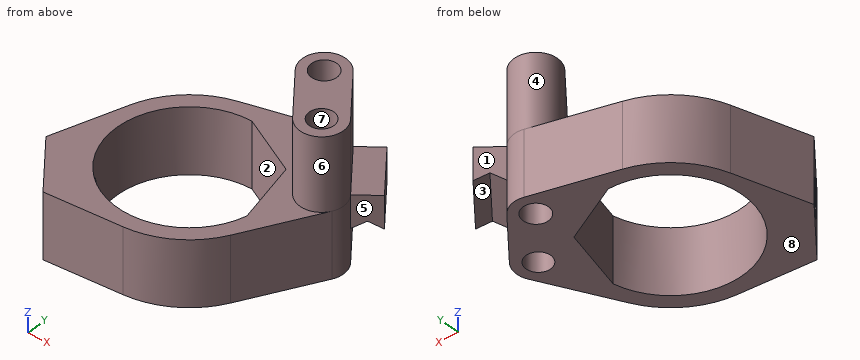
Autodesk Inventor part; units mm, degrees
ref_plane "YZ Plane" through (0, 0, 0) normal (1, 0, 0) x (0, 1, 0)
ref_plane "XZ Plane" through (0, 0, 0) normal (0, 1, 0) x (-1, 0, 0)
ref_plane "XY Plane" through (0, 0, 0) normal (0, 0, 1) x (1, 0, 0)
sketch "Sketch1" plane through (0, 0, 0) normal (0, 0, 1) x (1, 0, 0)
  circle A0 centre (83.2518, -42.1897) radius 1.5
  circle A1 centre (88.3962, -48.3162) radius 1.5
  circle A2 centre (75.2518, -54.1305) radius 10
  arc A3 (71.6612, -42.6802) -> (85.9084, -59.6473) centre (75.2518, -54.1305) ccw
  arc A4 (85.5492, -40.2605) -> (82.3541, -39.3271) centre (83.2518, -42.1897) ccw
  arc A5 (91.0604, -49.6954) -> (90.6937, -46.387) centre (88.3962, -48.3162) ccw
  line L0 (71.6612, -42.6802) -> (82.3541, -39.3271)
  line L1 (91.0604, -49.6954) -> (85.9084, -59.6473)
  line L2 (85.5492, -40.2605) -> (90.6937, -46.387)
  circle A6 centre (83.2518, -42.1897) radius 1.75
  circle A7 centre (88.3962, -48.3162) radius 1.7
  line L3 (88.1215, -43.3238) -> (66.062, -61.8472) construction
  line L4 (82.9099, -47.6999) -> (85.0453, -56.1521)
  line L5 (82.9099, -47.6999) -> (74.9544, -44.1349)
  circle A8 centre (75.2518, -54.1305) radius 9 construction
  line L6 (60.8256, -60.2763) -> (66.7035, -67.2763)
  line L7 (60.8256, -60.2763) -> (63.7758, -50.6232)
  line L8 (66.7035, -67.2763) -> (76.7214, -66.0401)
  point P0 (0, 0)
  dimension "d0" = 24
  dimension "d1" = 6
  dimension "d2" = 6
  dimension "d3" = 3.5
  dimension "d4" = 3.4
  dimension "d5" = 18
  dimension "d8" = 15
  dimension "d9" = 7
extrude "Extrusion1" add sketch "Sketch1" along normal blind 9 contours A2 L4 | L5 A2 | L0 A4 L2 A5 L1 A3 | A3 L8 L6 L7
sketch "Sketch2" plane through (66.7035, -67.2763, 0) normal (-0.7658175, -0.643058, 0) x (0, 0, 1)
  line L0 (9, 9.1406) -> (9, 0)
  line L1 (9, 4.5703) -> (0, 4.5703) construction
  line L2 (0, 9.1406) -> (0, 0)
  line L3 (0, 9.1406) -> (9, 9.1406)
  line L4 (4.5, 9.1406) -> (4.5, 0) construction
  line L5 (0, 0) -> (9, 0)
  point P0 (0, 94.4156)
  point P1 (4.5, 4.5703)
hole "Hole1" at (63.7645, -63.7763, 4.5) direction (0.7658175, 0.643058, 0) diameter 4.6 depth 8
ref_plane "Work Plane1" through (122.4886, -30.1352, -3.9205) normal (0.643058, -0.7658175, 0) x (0, 0, 1)
sketch "Sketch3" plane through (122.4886, -30.1352, -3.9205) normal (0.643058, -0.7658175, 0) x (0, 0, 1)
  line L0 (3.9205, 34.8) -> (12.9205, 34.8)
  line L1 (8.4716, 29.3) -> (8.4716, 32.8)
  line L2 (8.4716, 32.8) -> (8.4716, 33.3)
  line L3 (3.9205, 34.8) -> (12.9205, 34.8)
  line L4 (8.4716, 34.8) -> (9.4716, 33.05)
  line L5 (9.4716, 33.05) -> (8.4716, 31.3)
  line L6 (8.4716, 31.3) -> (12.9205, 31.3)
  line L7 (12.9205, 31.3) -> (12.9205, 34.8)
  line L8 (8.4716, 33.05) -> (10.4716, 33.05) construction
  point P0 (3.9205, 74.4253)
  dimension "d17" = 0.5
  dimension "d18" = 1
extrude "Extrusion2" add sketch "Sketch3" against normal blind 16
sketch "Sketch4" plane through (122.4886, -30.1352, -3.9205) normal (0.643058, -0.7658175, 0) x (0.7658175, 0.643058, 0)
  line L0 (-34.8, 12.9205) -> (-34.8, 8.4716)
  line L1 (-34.8, 8.4716) -> (-33.05, 9.4716)
  line L2 (-33.05, 9.4716) -> (-31.3, 8.4716)
  line L3 (-31.3, 8.4716) -> (-31.3, 12.9205)
  line L4 (-31.3, 12.9205) -> (-34.8, 12.9205)
  point P0 (-74.4253, 3.9205)
extrude "Extrusion3" cut sketch "Sketch4" against normal blind 8
sketch "Sketch5" plane through (0, 0, 9) normal (0, 0, 1) x (1, 0, 0)
  circle A0 centre (83.2518, -42.1897) radius 1.75
  circle A1 centre (83.2518, -42.1897) radius 1.75
  circle A2 centre (88.3962, -48.3162) radius 1.7
  circle A3 centre (88.3962, -48.3162) radius 1.7
  circle A4 centre (88.3962, -48.3162) radius 3
  circle A5 centre (83.2518, -42.1897) radius 3
  line L0 (85.5492, -40.2605) -> (90.6937, -46.387)
  line L1 (80.9543, -44.1188) -> (86.0988, -50.2454)
  point P0 (0, 0)
  dimension "d23" = 6
  dimension "d24" = 6
extrude "Extrusion4" add sketch "Sketch5" along normal blind 10
properties part number "marker_cerret"
CAD build for the part. Positions are in the model's coordinates, mm. Face numbers are marked on the shaded views. A direction names the side the tool comes from. Coordinates: 2 decimals unless noted, no trailing zeros. Write each loop counter-clockwise with the first axis right and the second up, starting at its lowest first coordinate (ties: lowest second). Pieces come first, ordered by that corner, then holes. Notation, with made-up numbers: M -30,-28.5 L 3,-28.5 A38 cw 3,10.5 Z; hole C 43.5,26.25 d6. An arc over 180 degrees is marked long. Answer as a JSON object with one key per item and string values. Group by question number.
1) Pin check, flat tips, straight feed: pin 1 Ø6 at (x, z) = (79.5, 4.5) entering from -Y; pin 2 Ø4 at (x, z) = (84, 10) entering from -Y; pin 3 Ø14 at (x, y) = (76.5, -51) entering from +Z; pin 4 Ø3 at (x, y) = (88.4, -48.32) entering from -Z. Stop position of each tip, or through.
2) Saw through at B-B (x = 77.5). Write the cut outline in (y, z).
3) Wall check: line 1 (Z direction, x = 85.5, y = -55.25); line 2 (X direction, y = -48.25, z = 7.5); line 3 (Y direction, x = 70, z = 1.5). Give the ranges that are in metal, low to high. Write a range as from..to.
4) Tool access for the marked faces 1, 2, 3, 4 and 5: list every direction of +Z, -Z, +X, -X, +Y, -Y with a clear straight run to the whole face (end or side of a thin tool).
5) Saw through at A-A (y = -52.75). Write the cut outline in (x, z), plus the area to 3 significant figures.
6) Saw through at D-D (z = 13.75). Write the cut outline in (x, y), plus the area to 3 significant figures.
7) Mould opens along Y. For the marked faces 6, 7 and 8 say: +Y half, -Y half, draft (parallel to the pull), parting line (faces both ways), or undercut.
8) Saw through at C-C (z = 1.5). Write the cut outline in (x, y), plus the area to 3 significant figures.
Values follow:
{
 "1": {"pin 1": "stops at y = -66.07", "pin 2": "stops at y = -63.87", "pin 3": "stops at z = 9", "pin 4": "passes through"},
 "2": {"outline": "M -65.92,0 L -63.87,0 L -63.87,9 L -65.92,9 Z; M -45.28,0 L -40.85,0 L -40.85,9 L -45.28,9 Z"},
 "3": {"line 1": "z = 0..9", "line 2": "x = 64.79..67.16, 83.05..86.7, 90.09..91.4", "line 3": "y = -66.87..-62.64, -45.62..-43.34"},
 "4": {"face 1": "+Z, -Z, +Y", "face 2": "+Z, -Z", "face 3": "-Z", "face 4": "+Z", "face 5": "+Z, -Z, +X"},
 "5": {"outline": "M 63.13,0 L 65.35,0 L 65.35,9 L 63.13,9 Z; M 84.19,0 L 89.48,0 L 89.48,9 L 84.19,9 Z", "area": "67.6 mm2"},
 "6": {"outline": "M 80.95,-44.12 L 86.1,-50.25 A3 ccw 90.69,-46.39 L 85.55,-40.26 A3 ccw Z; hole C 83.25,-42.19 d3.5; hole C 88.4,-48.32 d3.4", "area": "57.6 mm2"},
 "7": {"face 6": "parting line", "face 7": "undercut", "face 8": "draft"},
 "8": {"outline": "M 60.83,-60.28 L 66.7,-67.28 L 76.72,-66.04 A12 ccw 85.91,-59.65 L 91.06,-49.7 A3 ccw 90.69,-46.39 L 85.55,-40.26 A3 ccw 82.35,-39.33 L 71.66,-42.68 A12 ccw 63.78,-50.62 Z; hole M 74.95,-44.13 A10 ccw long 85.05,-56.15 L 82.91,-47.7 Z; hole C 83.25,-42.19 d3.5; hole C 88.4,-48.32 d3.4", "area": "266 mm2"}
}
